from build123d import *

# Parameters (mm, degrees)
BOSS_EXTRUDE1_DEPTH      = 11
BOSS_EXTRUDE1_DEPTH_BACK = 4
CUT_EXTRUDE1_OUTLINE_R   = 3.25
CUT_EXTRUDE1_DEPTH       = 10
CUT_EXTRUDE3_START       = -3.5
CUT_EXTRUDE3_OUTLINE_R   = 4.5
CUT_EXTRUDE3_DEPTH       = 1
CUT_EXTRUDE4_REACH       = 64.7
SKETCH5_R                = 3.75
CUT_EXTRUDE5_DEPTH       = 2.5
FILLET1_R                = 5
FILLET2_R                = 5
FILLET3_R                = 5
FILLET4_R                = 2
FILLET5_R                = 4
FILLET6_R                = 4


# Read off the part's stored shape, not the designer's step: Cut-Extrude1, Cut-Extrude3
with BuildPart() as part:
    # Sketch2 → Boss-Extrude1 (new, two sides: drawn at the far end of the back side and taken through both)
    with BuildSketch(Plane(origin=(0, 0, 0), x_dir=(1, 0, 0), z_dir=(0, 1, 0)).offset(-BOSS_EXTRUDE1_DEPTH_BACK)):
        Polygon((0, 5), (0, -22), (-3.5, -22), (-3.5, -60), (0, -60), (0, -35), (7, -35), (7, -7), (12, -7), (12, 5), align=None)
    extrude(amount=BOSS_EXTRUDE1_DEPTH + BOSS_EXTRUDE1_DEPTH_BACK)

    # Cut-Extrude1 outline → Cut-Extrude1 (cut)
    with BuildSketch(Plane.YZ):
        with Locations((3.5, 3.5)):
            Circle(CUT_EXTRUDE1_OUTLINE_R)
    extrude(amount=CUT_EXTRUDE1_DEPTH, mode=Mode.SUBTRACT)

    # Cut-Extrude3 outline → Cut-Extrude3 (cut)
    with BuildSketch(Plane.YZ.offset(CUT_EXTRUDE3_START)):
        with Locations((3.5, 50.074977824)):
            Circle(CUT_EXTRUDE3_OUTLINE_R)
    extrude(amount=CUT_EXTRUDE3_DEPTH, mode=Mode.SUBTRACT)

    # Sketch5 → Cut-Extrude4 (cut, up to next)
    with BuildSketch(Plane.ZY.offset(2.5), mode=Mode.PRIVATE) as cut_extrude4_sk1:
        with Locations((50.074977824, 3.5)):
            Circle(SKETCH5_R)
    cut_extrude4_tool1 = extrude(cut_extrude4_sk1.sketch, amount=-CUT_EXTRUDE4_REACH, mode=Mode.PRIVATE) & part.part
    add(cut_extrude4_tool1.solids().sort_by_distance((-2.5, 3.5, 50.074978))[0], mode=Mode.SUBTRACT)

    # Sketch10 → Cut-Extrude5 (cut)
    with BuildSketch(Plane.ZY.offset(3.5)):
        with BuildLine():
            ThreePointArc((41.962487455, 5), (41.859427156, 4.25314489), (41.824977824, 3.5))
            Line((41.824977824, 3.5), (42.824977824, 3.5))
            Line((42.824977824, 3.5), (42.824977824, 5))
            Line((42.824977824, 5), (41.962487455, 5))
        make_face()
        with BuildLine():
            Line((42.824977824, 3.5), (41.824977824, 3.5))
            ThreePointArc((41.824977824, 3.5), (41.859427156, 2.74685511), (41.962487455, 2))
            Line((41.962487455, 2), (42.824977824, 2))
            Line((42.824977824, 2), (42.824977824, 3.5))
        make_face()
    extrude(amount=-CUT_EXTRUDE5_DEPTH, mode=Mode.SUBTRACT)

    # Fillet1
    fillet1_edges = [part.edges().sort_by_distance(p)[0] for p in [
        (6, -4, -5),
        (6, 11, -5),
        (-1.75, -4, 60),
        (-1.75, 11, 60),
    ]]
    fillet(fillet1_edges, radius=FILLET1_R)

    # Fillet2
    # the kernel refuses this fillet: 5 mm, written as the material it takes off along each edge
    with BuildSketch(Plane(origin=(-3.5, -15.924240018, 22), x_dir=(1, 0, 0), z_dir=(0, 1, 0))) as fillet2_piece_1:
        with BuildLine():
            CenterArc((5, -4.769696007), FILLET2_R, 107.457603124, 72.542396876)
            Line((0, -4.769696007), (-0.1, -4.769696007))
            Line((-0.1, -4.769696007), (-0.1, 0))
            Line((-0.1, 0), (0, 0.1))
            ThreePointArc((0, 0.1), (1.75, 0.1), (3.47, 0.09539392))
            Line((3.47, 0.09539392), (3.5, 0))
        make_face()
    extrude(amount=38.848480035, mode=Mode.SUBTRACT)

    # Fillet3
    fillet3_edges = [part.edges().sort_by_distance(p)[0] for p in [
        (7, 3.5, 35),
    ]]
    fillet(fillet3_edges, radius=FILLET3_R)

    # Fillet4
    fillet4_edges = [part.edges().sort_by_distance(p)[0] for p in [
        (12, 3.5, 7),
    ]]
    fillet(fillet4_edges, radius=FILLET4_R)

    # Fillet5
    fillet5_edges = [part.edges().sort_by_distance(p)[0] for p in [
        (7, 3.5, 7),
        (0, 3.5, 35),
    ]]
    fillet(fillet5_edges, radius=FILLET5_R)

    # Fillet6
    fillet6_edges = [part.edges().sort_by_distance(p)[0] for p in [
        (0, 3.5, 22),
    ]]
    fillet(fillet6_edges, radius=FILLET6_R)


solid = part.part
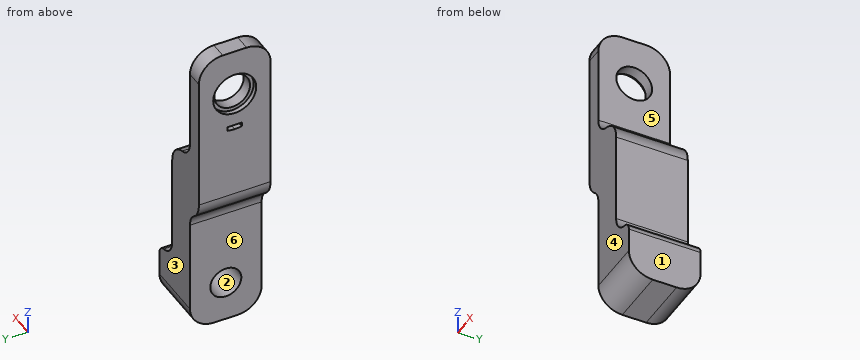
Part model, mm, in its own coordinate system. Face numbers are marked on the shaded views. A direction names the side the tool comes from. Give positions to 0.01 mm unless a question says otherwise; leave off trailing zeros. Loops run counter-clockwise (first coordinate to the right, second up) from the corner with the lowest first, then second, coordinate; pieces in that order, holes last. Notation, with made-up numbers: M 30.25,-12 L 48.25,-12 A21 cw 48.25,25 Z; hole C 80,28 d7. An arc over 180 degrees is marked long. Put each result on its own line as item: value. Start each with the question number.
1) 3-axis set-ups, long thin cutter, end or side, ignore diameter. For the marked faces 4, 5 and 6: which of +Z, -Z, +X, -X, +Y, -Y reach the whole face in a straight line?
2) Flat gauge pins, fed straight in: pin 1 (1 mm diameter, centred on x = 8.5, z = 33.5, fed in from +Y); pin 2 (1.2 mm diameter, centred on x = -2.5, y = 3, fed in from -Z); pin 3 (2 mm diameter, centred on y = 4, z = 4.5, fed in from -X); pin 4 (2 mm diameter, centred on y = 6.5, z = 15.5, fed in from -X). Where does each tip first touch, or does it go through?
3) Saw through at A-A (z = 3.5). List the corners of the cut face in (x, y), then the cut area to 3 significant figures.
4) Saw through at B-B (z = 16.5). List the corners of the cut face in (x, y), then the cut area to 3 significant figures.
5) Pull direction Y, two halves, no side cores. Call the marked faces 1, 2 and 3: +Y half, -Y half, draft (parallel to the pull), parting line (faces both ways), or undercut.
6) Probe probe 1 along Z at (x, y) = (-2.85, 3.5); probe 2 along Z at (x, y) = (-2.95, 3.5); probe 3 along X at (y, z) = (2.5, 57). List the from-to ranges inside material, lowest first.
Numbers:
1. face 4: +Z, -Z, +X, -X, -Y
1. face 5: +Z, +X, +Y, -Y
1. face 6: -Z, -X, +Y, -Y
2. pin 1: through
2. pin 2: z = 23.1
2. pin 3: x = 10
2. pin 4: x = 0
3. outline: M 0,-4 L 12,-4 L 12,11 L 0,11 L 0,6.75 L 10,6.75 L 10,0.25 L 0,0.25 Z
3. area: 115 mm^2
4. outline: M 0,-4 L 7,-4 L 7,11 L 0,11 Z
4. area: 105 mm^2
5. face 1: draft
5. face 2: undercut
5. face 3: +Y half
6. probe 1: 24.3 to 41.82, 42.82 to 45.57, 54.57 to 60
6. probe 2: 24.49 to 41.82, 42.82 to 45.57, 54.57 to 60
6. probe 3: -3.5 to 0
